For this review, take the finished solid that the model builds, in its own axes (mm). Face numbers are marked on the shaded views. A direction names the side the tool comes from. Round coordinates to 2 decimals unless told otherwise and drop trailing zeros. Order: outer loops, then holes, each group sorted by start corner. A loop starts at its lowest first (then second) coordinate and runs counter-clockwise, first axis right, second up. Notation, with made-up numbers: M 10,22.5 L 29,22.5 A21 cw 29,39.5 Z; hole C 34,38.5 d11. An arc over 180 degrees is marked long. Answer as a JSON object with one key per item and string values.
from build123d import *

# Parameters (mm, degrees)
F1_DEPTH = 10
F2_T     = -1


with BuildPart() as f1:
    # F0 (on Top) → F1 (new body)
    with BuildSketch(Plane.XY):
        with BuildLine():
            Line((-90, 75), (-90, 15))
            ThreePointArc((-90, 15), (-85.606602, 4.393398), (-75, 0))
            ThreePointArc((-75, 0), (-64.393398, 4.393398), (-60, 15))
            Line((-60, 15), (-60, 45))
            ThreePointArc((-60, 45), (-55.606602, 55.606602), (-45, 60))
            ThreePointArc((-45, 60), (-34.393398, 55.606602), (-30, 45))
            Line((-30, 45), (-30, 15))
            ThreePointArc((-30, 15), (-25.606602, 4.393398), (-15, 0))
            ThreePointArc((-15, 0), (-4.393398, 4.393398), (0, 15))
            Line((0, 15), (0, 75))
            ThreePointArc((0, 75), (-4.393398, 85.606602), (-15, 90))
            Line((-15, 90), (-75, 90))
            ThreePointArc((-75, 90), (-85.606602, 85.606602), (-90, 75))
        make_face()
    extrude(amount=F1_DEPTH)

    # F2
    f2_openings = [f1.faces().sort_by_distance(p)[0] for p in [
        (-5.293398, 84.706602, 10),
    ]]
    offset(amount=F2_T, openings=f2_openings)


solid = f1.part
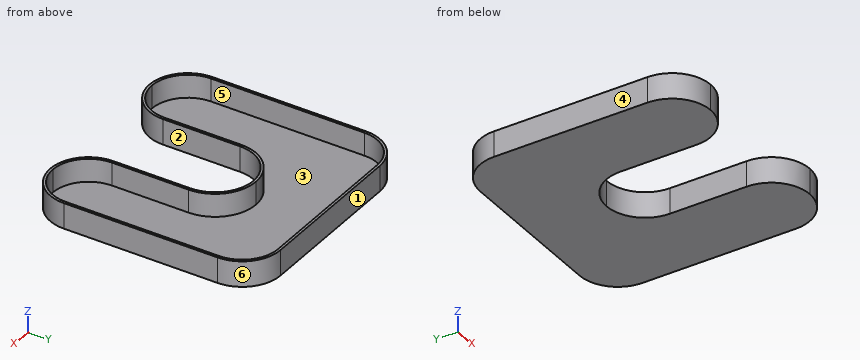
1) Add section C-C on x = -79. State the section outline as (y, z) points, and give its area (3 significant figures).
Geometry check:
{"outline": "M 0.54,0 L 89.46,0 L 89.46,10 L 88.42,10 L 88.42,1 L 1.58,1 L 1.58,10 L 0.54,10 Z", "area": "108 mm²"}
2) Add section D-D on y = 49. State the section outline as (x, z) points, and give its area (3 significant figures).
Geometry check:
{"outline": "M -90,0 L -59.46,0 L -59.46,10 L -60.49,10 L -60.49,1 L -89,1 L -89,10 L -90,10 Z; M -30.54,0 L 0,0 L 0,10 L -1,10 L -1,1 L -29.51,1 L -29.51,10 L -30.54,10 Z", "area": "97.7 mm²"}
3) Add section A-A on y = 18.5. State the section outline as (x, z) points.
Geometry check:
{"outline": "M -90,0 L -60,0 L -60,10 L -61,10 L -61,1 L -89,1 L -89,10 L -90,10 Z; M -30,0 L 0,0 L 0,10 L -1,10 L -1,1 L -29,1 L -29,10 L -30,10 Z"}
4) Machinability: for the marked faces 1, 2 and 3, which of the approach directions +Z, -Z, +X, -X, +Y, -Y give a long, thin tool a straight path to every point of the face, cutting with its end or side? Answer none if there is none.
Geometry check:
{"face 1": "+Z, -Z, +X, -X, +Y", "face 2": "+Z, -Z, -Y", "face 3": "+Z"}
5) For L1, parallel to X at y = 20, z = 4.25; L2, parallel to X at y = 58, z = 9.25; L3, parallel to Y at x = -75.5, z = 9.5, list the stretches that pass through material, from the lowest coordinate up.
Geometry check:
{"L1": "x = -90 to -89, -61 to -60, -30 to -29, -1 to 0", "L2": "x = -90 to -89, -54.33 to -52.48, -37.52 to -35.67, -1 to 0", "L3": "y = 0.01 to 1.01, 88.99 to 89.99"}
6) Mouldability with a two-part tool opening along Y and no side actions: class the marked faces 4, 5 and 6 as +Y half, -Y half, draft (parallel to the pull), parting line (faces both ways), or undercut.
Geometry check:
{"face 4": "draft", "face 5": "undercut", "face 6": "+Y half"}
7) Insertion check: P1, Ø3, axis at x = -19, y = 80, coming from the +Z side; P2, Ø1.5, axis at x = -33, z = 8, coming from the -Y side. Each pin has a flat end and moves straight along its axis. Give the tip position at first contact, or say it passes through.
Geometry check:
{"P1": "stops at z = 1", "P2": "stops at y = 52.9"}
8) Add section B-B on z = 8.75. State the section outline as (x, y) points.
Geometry check:
{"outline": "M -90,15 A15 ccw -75,0 A15 ccw -60,15 L -60,45 A15 cw -45,60 A15 cw -30,45 L -30,15 A15 ccw -15,0 A15 ccw 0,15 L 0,75 A15 ccw -15,90 L -75,90 A15 ccw -90,75 Z; hole M -89,15 A14 ccw -75,1 A14 ccw -61,15 L -61,45 A16 cw -45,61 A16 cw -29,45 L -29,15 A14 ccw -15,1 A14 ccw -1,15 L -1,75 A14 ccw -15,89 L -75,89 A14 ccw -89,75 Z"}
